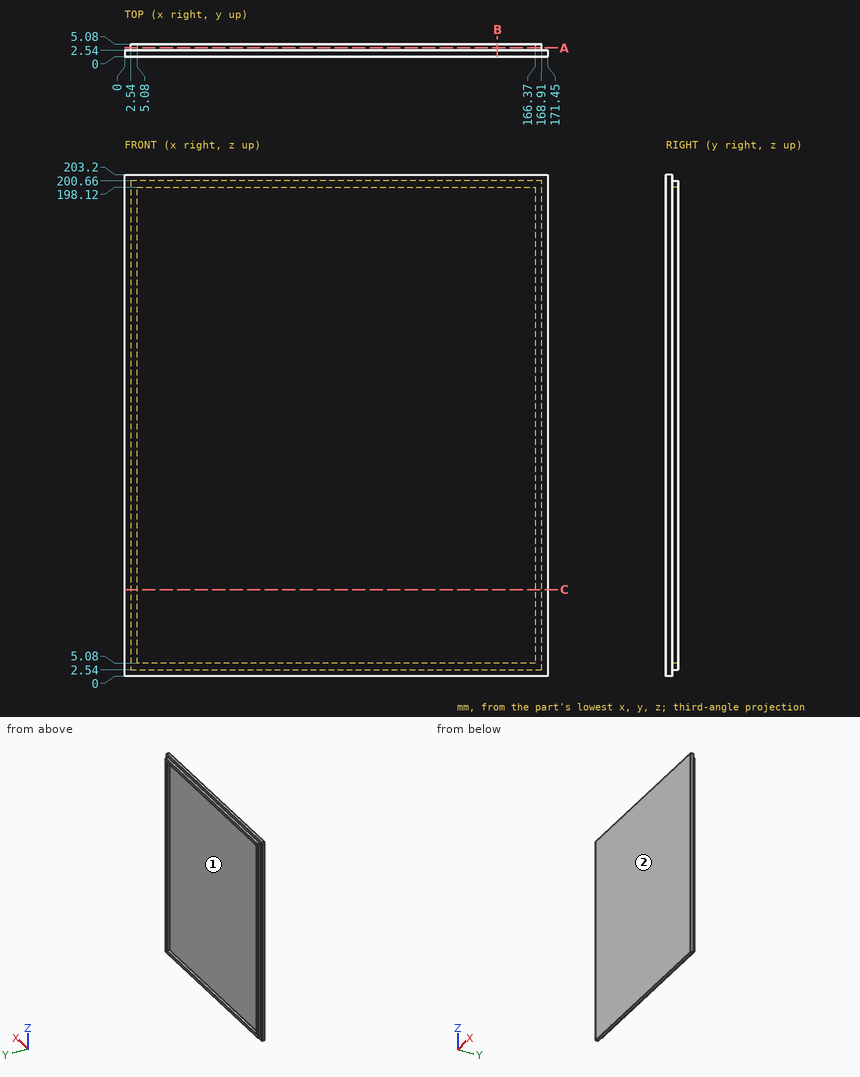
For this review, use the dimensioned drawing (mm, ordinates from the lowest corner) and the shaded views. Round coordinates to 2 decimals unless told otherwise and drop trailing zeros. Loops run counter-clockwise (first coordinate to the right, second up) from the corner with the lowest first, then second, coordinate; pieces in that order, holes last. Notation, with made-up numbers: M -3.75,-19 L 40.25,-19 A16 ccw 40.25,-5 Z; hole C 84.5,47.25 d1. An arc over 180 degrees is marked long. Answer as CSV lines item,"result".
1. We need section C-C (z = 35). Give the boundary of the cut face in (x, y), plus the area to 3 significant figures.
Outcome:
outline,"M 0,0 L 171.45,0 L 171.45,2.54 L 168.91,2.54 L 168.91,5.08 L 166.37,5.08 L 166.37,2.54 L 5.08,2.54 L 5.08,5.08 L 2.54,5.08 L 2.54,2.54 L 0,2.54 Z"
area,"448 mm2"
2. We need section A-A (y = 3.55). Give the boundary of the cut face in (x, z), plus the area to 3 significant figures.
Outcome:
outline,"M 2.54,2.54 L 168.91,2.54 L 168.91,200.66 L 2.54,200.66 Z; hole M 5.08,5.08 L 166.37,5.08 L 166.37,198.12 L 5.08,198.12 Z"
area,"1,830 mm2"
3. Draft analysis for pull direction Z (two halves, no side actions). For the marked faces 1 and 2, state which applies: pulls with the +Z half, pulls with the -Z half, needs draft (parallel to the pull), parting line crosses it, or undercut.
Outcome:
face 1,"undercut"
face 2,"needs draft"
4. Insertion check: pin 1 Ø1.3 at (x, y) = (125, 4) entering from -Z; pin 2 Ø1.5 at (x, z) = (69, 82) entering from +Y; pin 3 Ø1.3 at (y, z) = (4, 138.5) entering from +X. Each pin has a flat end and moves straight along its axis. Give the tip position at first contact, or say it passes through.
Outcome:
pin 1,"stops at z = 2.54"
pin 2,"stops at y = 2.54"
pin 3,"stops at x = 168.91"
5. To check wall thickness, follow L1, parallel to X at y = 4.3, z = 185; L2, parallel to Z at x = 12, y = 2.95; L3, parallel to Y at x = 111, z = 33. State the ranges of each line that lie inside material, in increasing order. Write a range as [from, to].
Outcome:
L1,"x = [2.54, 5.08], [166.37, 168.91]"
L2,"z = [2.54, 5.08], [198.12, 200.66]"
L3,"y = [0, 2.54]"
6. We need section B-B (x = 151). Give the boundary of the cut face in (y, z).
Outcome:
outline,"M 0,0 L 2.54,0 L 2.54,2.54 L 5.08,2.54 L 5.08,5.08 L 2.54,5.08 L 2.54,198.12 L 5.08,198.12 L 5.08,200.66 L 2.54,200.66 L 2.54,203.2 L 0,203.2 Z"
